Verification items for this drawing (mm, ordinates from the low corner). Coordinates: 2 decimals unless noted, no trailing zeros. Order: outer loops, then holes, each group sorted by start corner. A loop starts at its lowest first (then second) coordinate and runs counter-clockwise, first axis right, second up.
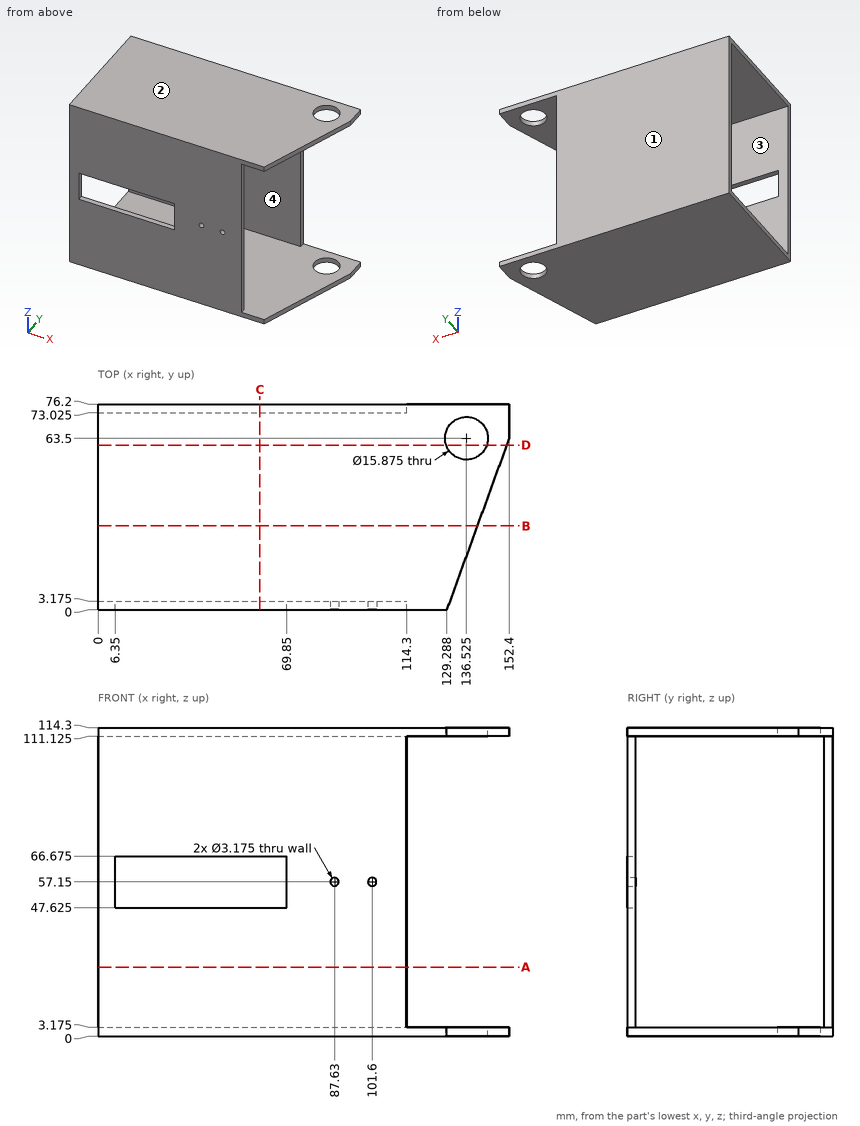
(1) Cross-section at D-D (y = 61). Enter the section's corners in (x, z) (1 decimal), and give its area (3 significant figures).
Filled in:
outline: (0, 0) - (129, 0) - (129, 3.2) - (0, 3.2) - close; (0, 111.1) - (129, 111.1) - (129, 114.3) - (0, 114.3) - close; (144.1, 0) - (151.5, 0) - (151.5, 3.2) - (144.1, 3.2) - close; (144.1, 111.1) - (151.5, 111.1) - (151.5, 114.3) - (144.1, 114.3) - close
area: 866 mm2
(2) Cross-section at C-C (x = 60). Enter the section's corners in (y, z) (3 decimals), and give its area (3 significant figures).
Filled in:
outline: (0, 0) - (76.2, 0) - (76.2, 114.3) - (0, 114.3) - (0, 66.675) - (3.175, 66.675) - (3.175, 111.125) - (73.025, 111.125) - (73.025, 3.175) - (3.175, 3.175) - (3.175, 47.625) - (0, 47.625) - close
area: 1,110 mm2
(3) Cross-section at B-B (y = 31). Enter the section's corners in (x, z) (3 decimals).
Filled in:
outline: (0, 0) - (140.571, 0) - (140.571, 3.175) - (0, 3.175) - close; (0, 111.125) - (140.571, 111.125) - (140.571, 114.3) - (0, 114.3) - close
(4) Go/stop test with a flat-tipped pin: P1, Ø1.6, axis at y = 1, z = 48, coming from the +X side. Record where the tip stops, or that it passes through.
Filled in:
P1: stops at x = 114.3
(5) Release check for a two-part mould opening along Z. For the marked faces 1, 2, 3 and 4 record: +Z half, -Z half, draft (parallel to the pull), parting line (faces both ways), or undercut.
Filled in:
face 1: draft
face 2: +Z half
face 3: undercut
face 4: undercut
(6) Thickness scan on probe 1 along Z at (x, y) = (52, 47) (3 decimals); probe 2 along Y at (x, z) = (57, 43) (3 decimals); probe 3 along X at (y, z) = (63.5, 2). Record the ranges inside material, lowest first.
Filled in:
probe 1: z = 0 to 3.175, 111.125 to 114.3
probe 2: y = 0 to 3.175, 73.025 to 76.2
probe 3: x = 0 to 128.59, 144.46 to 152.4
(7) Cross-section at A-A (z = 25.5). Enter the section's corners in (x, y) (3 decimals), and give its area (3 significant figures).
Filled in:
outline: (0, 0) - (114.3, 0) - (114.3, 3.175) - (0, 3.175) - close; (0, 73.025) - (114.3, 73.025) - (114.3, 76.2) - (0, 76.2) - close
area: 726 mm2
